Check sheet for the modelled part. Datum: model origin and axes. Units: mm. Round coordinates to 2 decimals unless told otherwise and drop trailing zeros. Order: outer loops, then holes, each group sorted by start corner. A loop starts at its lowest first (then second) coordinate and runs counter-clockwise, first axis right, second up.
Q1. Depth check by flat-ended pin: P1, Ø7, axis at y = -1, z = 321.5, coming from the +X side; P2, Ø3, axis at x = -2, z = 307.5, coming from the +Y side; P3, Ø1.5, axis at x = 0.5, z = 294, coming from the -Y side. Enter the tip coordinate at first touch or a pass-through.
Q2. Cross-section at A-A on y = 0. Record the cut outline in (x, z).
Q3. Scan lines: probe 1 along Y at (x, z) = (6.5, 289.5); probe 2 along Y at (x, z) = (0, 336.5); probe 3 along X at (y, z) = (9, 340.5). Record each from-to range of solid material in increasing order.
from build123d import *

# Parameters (mm, degrees)
SKETCH1_R               = 3.4036
BOSS_EXTRUDE1_DEPTH     = 380
SKETCH2_W               = 379
SKETCH2_H               = 40
CUT_EXTRUDE1_DEPTH      = 65
CUT_EXTRUDE1_DEPTH_BACK = 71
SKETCH4_W               = 279.4
SKETCH4_H               = 55.537742005
CUT_EXTRUDE2_DEPTH      = 30
CUT_EXTRUDE2_DEPTH_BACK = 30


with BuildPart() as part:
    # Sketch1 → Boss-Extrude1 (new body, symmetric)
    with BuildSketch(Plane.XY):
        with BuildLine():
            Line((-20, 16.952), (-20, 4.7625))
            ThreePointArc((-20, 4.7625), (-19.776815367, 4.223684633), (-19.238, 4.0005))
            Line((-19.238, 4.0005), (-16.2662, 4.0005))
            ThreePointArc((-16.2662, 4.0005), (-15.727384633, 4.223684633), (-15.5042, 4.7625))
            Line((-15.5042, 4.7625), (-15.5042, 10.2235))
            ThreePointArc((-15.5042, 10.2235), (-15.033804775, 10.927496204), (-14.203384633, 10.762315367))
            Line((-14.203384633, 10.762315367), (-8.635059555, 5.19399029))
            ThreePointArc((-8.635059555, 5.19399029), (-7.985348265, 4.221628629), (-7.7572, 3.074649845))
            Line((-7.7572, 3.074649845), (-7.7572, -3.074649845))
            ThreePointArc((-7.7572, -3.074649845), (-7.985348265, -4.221628629), (-8.635059555, -5.19399029))
            Line((-8.635059555, -5.19399029), (-14.203384633, -10.762315367))
            ThreePointArc((-14.203384633, -10.762315367), (-15.033804775, -10.927496204), (-15.5042, -10.2235))
            Line((-15.5042, -10.2235), (-15.5042, -4.7625))
            ThreePointArc((-15.5042, -4.7625), (-15.727384633, -4.223684633), (-16.2662, -4.0005))
            Line((-16.2662, -4.0005), (-19.238, -4.0005))
            ThreePointArc((-19.238, -4.0005), (-19.776815367, -4.223684633), (-20, -4.7625))
            Line((-20, -4.7625), (-20, -16.952))
            ThreePointArc((-20, -16.952), (-19.107261469, -19.107261469), (-16.952, -20))
            Line((-16.952, -20), (-4.7625, -20))
            ThreePointArc((-4.7625, -20), (-4.223684633, -19.776815367), (-4.0005, -19.238))
            Line((-4.0005, -19.238), (-4.0005, -16.2662))
            ThreePointArc((-4.0005, -16.2662), (-4.223684633, -15.727384633), (-4.7625, -15.5042))
            Line((-4.7625, -15.5042), (-10.2235, -15.5042))
            ThreePointArc((-10.2235, -15.5042), (-10.927496204, -15.033804775), (-10.762315367, -14.203384633))
            Line((-10.762315367, -14.203384633), (-5.19399029, -8.635059555))
            ThreePointArc((-5.19399029, -8.635059555), (-4.221628629, -7.985348265), (-3.074649845, -7.7572))
            Line((-3.074649845, -7.7572), (3.074649845, -7.7572))
            ThreePointArc((3.074649845, -7.7572), (4.221628629, -7.985348265), (5.19399029, -8.635059555))
            Line((5.19399029, -8.635059555), (10.762315367, -14.203384633))
            ThreePointArc((10.762315367, -14.203384633), (10.927496204, -15.033804775), (10.2235, -15.5042))
            Line((10.2235, -15.5042), (4.7625, -15.5042))
            ThreePointArc((4.7625, -15.5042), (4.223684633, -15.727384633), (4.0005, -16.2662))
            Line((4.0005, -16.2662), (4.0005, -19.238))
            ThreePointArc((4.0005, -19.238), (4.223684633, -19.776815367), (4.7625, -20))
            Line((4.7625, -20), (16.952, -20))
            ThreePointArc((16.952, -20), (19.107261469, -19.107261469), (20, -16.952))
            Line((20, -16.952), (20, -4.7625))
            ThreePointArc((20, -4.7625), (19.776815367, -4.223684633), (19.238, -4.0005))
            Line((19.238, -4.0005), (16.2662, -4.0005))
            ThreePointArc((16.2662, -4.0005), (15.727384633, -4.223684633), (15.5042, -4.7625))
            Line((15.5042, -4.7625), (15.5042, -10.2235))
            ThreePointArc((15.5042, -10.2235), (15.033804775, -10.927496204), (14.203384633, -10.762315367))
            Line((14.203384633, -10.762315367), (8.635059555, -5.19399029))
            ThreePointArc((8.635059555, -5.19399029), (7.985348265, -4.221628629), (7.7572, -3.074649845))
            Line((7.7572, -3.074649845), (7.7572, 3.074649845))
            ThreePointArc((7.7572, 3.074649845), (7.985348265, 4.221628629), (8.635059555, 5.19399029))
            Line((8.635059555, 5.19399029), (14.203384633, 10.762315367))
            ThreePointArc((14.203384633, 10.762315367), (15.033804775, 10.927496204), (15.5042, 10.2235))
            Line((15.5042, 10.2235), (15.5042, 4.7625))
            ThreePointArc((15.5042, 4.7625), (15.727384633, 4.223684633), (16.2662, 4.0005))
            Line((16.2662, 4.0005), (19.238, 4.0005))
            ThreePointArc((19.238, 4.0005), (19.776815367, 4.223684633), (20, 4.7625))
            Line((20, 4.7625), (20, 16.952))
            ThreePointArc((20, 16.952), (19.107261469, 19.107261469), (16.952, 20))
            Line((16.952, 20), (4.7625, 20))
            ThreePointArc((4.7625, 20), (4.223684633, 19.776815367), (4.0005, 19.238))
            Line((4.0005, 19.238), (4.0005, 16.2662))
            ThreePointArc((4.0005, 16.2662), (4.223684633, 15.727384633), (4.7625, 15.5042))
            Line((4.7625, 15.5042), (10.2235, 15.5042))
            ThreePointArc((10.2235, 15.5042), (10.927496204, 15.033804775), (10.762315367, 14.203384633))
            Line((10.762315367, 14.203384633), (5.19399029, 8.635059555))
            ThreePointArc((5.19399029, 8.635059555), (4.221628629, 7.985348265), (3.074649845, 7.7572))
            Line((3.074649845, 7.7572), (-3.074649845, 7.7572))
            ThreePointArc((-3.074649845, 7.7572), (-4.221628629, 7.985348265), (-5.19399029, 8.635059555))
            Line((-5.19399029, 8.635059555), (-10.762315367, 14.203384633))
            ThreePointArc((-10.762315367, 14.203384633), (-10.927496204, 15.033804775), (-10.2235, 15.5042))
            Line((-10.2235, 15.5042), (-4.7625, 15.5042))
            ThreePointArc((-4.7625, 15.5042), (-4.223684633, 15.727384633), (-4.0005, 16.2662))
            Line((-4.0005, 16.2662), (-4.0005, 19.238))
            ThreePointArc((-4.0005, 19.238), (-4.223684633, 19.776815367), (-4.7625, 20))
            Line((-4.7625, 20), (-16.952, 20))
            ThreePointArc((-16.952, 20), (-19.107261469, 19.107261469), (-20, 16.952))
        make_face()
        Circle(SKETCH1_R, mode=Mode.SUBTRACT)
    extrude(amount=BOSS_EXTRUDE1_DEPTH, both=True)

    # Sketch2 → Cut-Extrude1 (cut, two sides)
    with BuildSketch(Plane(origin=(0, 0, 0), x_dir=(0, 0, -1), z_dir=(1, 0, 0))) as cut_extrude1_sk:
        with Locations((190.5, 0)):
            Rectangle(SKETCH2_W, SKETCH2_H)
    extrude(amount=CUT_EXTRUDE1_DEPTH, mode=Mode.SUBTRACT)
    extrude(cut_extrude1_sk.sketch, amount=-CUT_EXTRUDE1_DEPTH_BACK, mode=Mode.SUBTRACT)

    # Sketch4 → Cut-Extrude2 (cut, two sides)
    with BuildSketch(Plane(origin=(0, 0, 0), x_dir=(0, 0, -1), z_dir=(1, 0, 0))) as cut_extrude2_sk:
        with Locations((-138.7, -7.768871003)):
            Rectangle(SKETCH4_W, SKETCH4_H)
    extrude(amount=CUT_EXTRUDE2_DEPTH, mode=Mode.SUBTRACT)
    extrude(cut_extrude2_sk.sketch, amount=-CUT_EXTRUDE2_DEPTH_BACK, mode=Mode.SUBTRACT)


solid = part.part
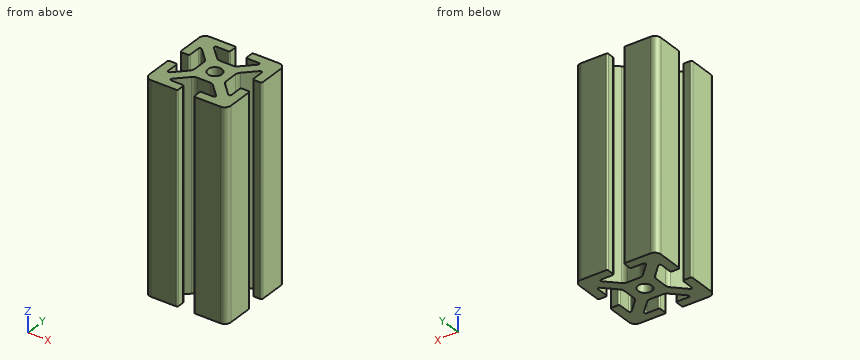
Results found:
1. P1: stops at x = 19.95
1. P2: stops at y = 7.79
1. P3: stops at y = -7.76
2. outline: (-7.76, 278.4) - (-3.4, 278.4) - (-3.4, 380) - (-7.76, 380) - close; (3.4, 278.4) - (7.76, 278.4) - (7.76, 380) - (3.4, 380) - close
3. probe 1: y = -20 to -15.5, -9.94 to 9.94, 15.5 to 20
3. probe 2: y = -7.76 to -3.4, 3.4 to 7.76
3. probe 3: x = -20 to -15.5, -12.44 to -5.56, 5.56 to 12.44, 15.5 to 20
